```python
from build123d import *

# Parameters (mm, degrees)
SKETCH1_R           = 57.5
BOSS_EXTRUDE1_DEPTH = 280
FILLET1_R           = 40
SKETCH2_R           = 13.5
BOSS_EXTRUDE2_DEPTH = 10
SKETCH3_R           = 15.5
BOSS_EXTRUDE3_DEPTH = 24
FILLET2_R           = 10
FILLET3_R           = 10


with BuildPart() as part:
    # Sketch1 → Boss-Extrude1 (new body)
    with BuildSketch(Plane.XY):
        Circle(SKETCH1_R)
    extrude(amount=BOSS_EXTRUDE1_DEPTH)

    # Fillet1
    fillet1_edges = [part.edges().sort_by_distance(p)[0] for p in [
        (-57.5, 0, 280),
    ]]
    fillet(fillet1_edges, radius=FILLET1_R)

    # Sketch2 → Boss-Extrude2 (add)
    with BuildSketch(Plane.XY.offset(280)):
        Circle(SKETCH2_R)
    extrude(amount=BOSS_EXTRUDE2_DEPTH)

    # Sketch3 → Boss-Extrude3 (add)
    with BuildSketch(Plane.XY.offset(290)):
        Circle(SKETCH3_R)
    extrude(amount=BOSS_EXTRUDE3_DEPTH)

    # Fillet2
    fillet2_edges = [part.edges().sort_by_distance(p)[0] for p in [
        (-13.5, 0, 280),
    ]]
    fillet(fillet2_edges, radius=FILLET2_R - 0.0001)  # a hair under: the kernel refuses the full size

    # Fillet3
    fillet3_edges = [part.edges().sort_by_distance(p)[0] for p in [
        (-57.5, 0, 0),
    ]]
    fillet(fillet3_edges, radius=FILLET3_R)


solid = part.part
```
Read the model definition and answer for the solid it produces. Units are mm, in the model's axes. A direction names the side the tool comes from. Give positions to 0.01 mm unless a question says otherwise; leave off trailing zeros. Loops run counter-clockwise (first coordinate to the right, second up) from the corner with the lowest first, then second, coordinate; pieces in that order, holes last.
Item 1: For faces 4 (the cylindrical face through (12.47, -5.17, 289.82)), 5 (the cylindrical face through (-2.018, 15.368, 301.832)), 6 (the cylindrical face through (-12.465, -56.133, 123.39)), determine the directions among +Z, -Z, +X, -X, +Y, -Y from which every point of the face is accessible in a straight line to the end or side of a thin tool.
Item 2: Each of these flat-tipped pins is pushed along its axis until it touches: pin 1 Ø1.5 at (x, y) = (-31, -42) entering from +Z; pin 2 Ø4 at (x, z) = (-43.5, 248) entering from -Y; pin 3 Ø2 at (y, z) = (24, 156) entering from +X. Where does it stop, or does it pass through?
Item 3: Find the intervals of material crossed by line 1 along Y through (x, z) = (53, 44); line 2 along X through (y, z) = (-44, 249); line 3 along Y through (x, z) = (11, 58.5), in increasing order.
Item 4: The mould has two halves that part along Z. Classify faces 1 (the flat face through (-1, 1, 0)), 2 (the flat face through (-5, 13, 290)), 3 (the flat face through (0, 0, 314)): released by +Z, released by -Z, zero draft, split by the parting line, or undercut.
Item 5: The part is cut by section A-A (z = 84). Write down the section's boundary in (x, y).
Taken from the geometry:
1. face 4: none
1. face 5: +Z
1. face 6: +Z, -Z
2. pin 1: stops at z = 261.15
2. pin 2: stops at y = -38.7
2. pin 3: stops at x = 52.7
3. line 1: y = -22.3 to 22.3
3. line 2: x = -35.4 to 35.4
3. line 3: y = -56.44 to 56.44
4. face 1: released by -Z
4. face 2: undercut
4. face 3: released by +Z
5. outline: circle Ø115 at (0, 0)
